Build history of the part. All positions in model axes, mm. A direction names the side the tool comes from. Give positions to 0.01 mm unless a question says otherwise; leave off trailing zeros. Write each loop counter-clockwise with the first axis right and the second up, starting at its lowest first coordinate (ties: lowest second). Pieces come first, ordered by that corner, then holes.
from build123d import *

# Parameters (mm, degrees)
CROQUIS1_R              = 23.9
CROQUIS1_R_2            = 8.45
SALIENTE_EXTRUIR1_DEPTH = 5
CROQUIS1_3_R            = 30
CROQUIS1_3_R_2          = 23.9
CROQUIS1_3_R_3          = 8.45
SALIENTE_EXTRUIR2_DEPTH = 5
CROQUIS2_R              = 20
CORTAR_EXTRUIR1_DEPTH   = 2


with BuildPart() as part:
    # Croquis1 → Saliente-Extruir1 (new body)
    with BuildSketch(Plane(origin=(0, 0, 0), x_dir=(1, 0, 0), z_dir=(0, 1, 0))):
        Circle(CROQUIS1_R)
        Circle(CROQUIS1_R_2, mode=Mode.SUBTRACT)
    extrude(amount=SALIENTE_EXTRUIR1_DEPTH)

    # Croquis1_3 → Saliente-Extruir2 (add)
    with BuildSketch(Plane(origin=(0, 0, 0), x_dir=(1, 0, 0), z_dir=(0, 1, 0))):
        Circle(CROQUIS1_3_R)
        Circle(CROQUIS1_3_R_2, mode=Mode.SUBTRACT)
        Circle(CROQUIS1_3_R_2)
        Circle(CROQUIS1_3_R_3, mode=Mode.SUBTRACT)
    extrude(amount=-SALIENTE_EXTRUIR2_DEPTH)

    # Croquis2 → Cortar-Extruir1 (cut)
    with BuildSketch(Plane(origin=(0, 5, 0), x_dir=(1, 0, 0), z_dir=(0, 1, 0))):
        Circle(CROQUIS2_R)
    extrude(amount=-CORTAR_EXTRUIR1_DEPTH, mode=Mode.SUBTRACT)


solid = part.part
(1) Drop flat-ended pins along their axis: pin 1 (1.5 mm diameter, centred on x = -9.5, y = -1, fed in from +Z); pin 2 (18 mm diameter, centred on x = 5, z = 2, fed in from +Y); pin 3 (1 mm diameter, centred on x = -12, y = 3.5, fed in from -Z); pin 4 (15 mm diameter, centred on x = 0, z = 0, fed in from +Y). Give the stop position or say it passes through.
(2) Probe line 1 (Z direction, x = 0, y = -1.5); line 2 (X direction, y = 1, z = 0); line 3 (X direction, y = 3.95, z = 0). List the from-to ranges inside material, lowest first.
(3) Mould opens along Z. For faces 1 (the face through (0, 3, 9)), 2 (the face through (6.2, -5, 6.2)), 3 (the face through (-29.97, -2.46, -1.32)) say: +Z half, -Z half, draft (parallel to the pull), parting line (faces both ways), or undercut.
(4) Saw through at D-D, the plane x = 14.5. List the corners of the cut face in (y, z).
(5) Saw through at A-A, the plane z = 0. List the corners of the cut face in (x, y).
(6) Saw through at B-B, the plane x = 0. List the corners of the cut face in (y, z), plus the area to 3 significant figures.
(7) 3-axis set-ups, long thin cutter, end or side, ignore diameter. For faces 4 (the face through (8.06, -0.94, -2.54)), 5 (the face through (-20.14, 0, 13.19)): which of +Z, -Z, +X, -X, +Y, -Y reach the whole face in a straight line?
(8) Saw through at C-C, the plane y = -1.25. List the corners of the cut face in (x, z), plus the area to 3 significant figures.
Computed values:
1. pin 1: stops at z = 28.7
1. pin 2: stops at y = 3
1. pin 3: stops at z = -20.95
1. pin 4: passes through
2. line 1: z = -30 to -8.45, 8.45 to 30
2. line 2: x = -23.9 to -8.45, 8.45 to 23.9
2. line 3: x = -23.9 to -20, 20 to 23.9
3. face 1: undercut
3. face 2: draft
3. face 3: parting line
4. outline: (-5, -26.26) - (0, -26.26) - (0, -19) - (5, -19) - (5, -13.77) - (3, -13.77) - (3, 13.77) - (5, 13.77) - (5, 19) - (0, 19) - (0, 26.26) - (-5, 26.26) - close
5. outline: (-30, -5) - (-8.45, -5) - (-8.45, 3) - (-20, 3) - (-20, 5) - (-23.9, 5) - (-23.9, 0) - (-30, 0) - close; (8.45, -5) - (30, -5) - (30, 0) - (23.9, 0) - (23.9, 5) - (20, 5) - (20, 3) - (8.45, 3) - close
6. outline: (-5, -30) - (0, -30) - (0, -23.9) - (5, -23.9) - (5, -20) - (3, -20) - (3, -8.45) - (-5, -8.45) - close; (-5, 8.45) - (3, 8.45) - (3, 20) - (5, 20) - (5, 23.9) - (0, 23.9) - (0, 30) - (-5, 30) - close
6. area: 324 mm2
7. face 4: +Y, -Y
7. face 5: +Y
8. outline: circle Ø60 at (0, 0); hole circle Ø16.9 at (0, 0)
8. area: 2,600 mm2
